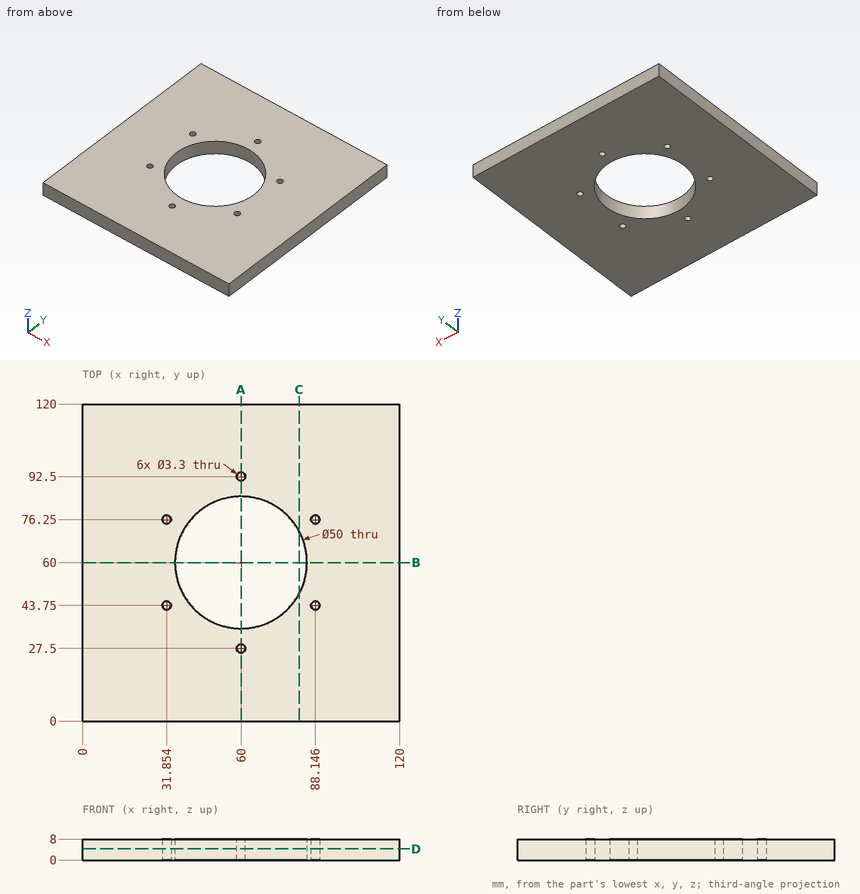
Here's the drawing with two shaded views (mm, measured from the low corner). I have some questions. Give positions to 0.01 mm unless a question says otherwise; leave off trailing zeros. Loops run counter-clockwise (first coordinate to the right, second up) from the corner with the lowest first, then second, coordinate; pieces in that order, holes last. Notation, with made-up numbers: M -9.75,78.25 L 30.25,78.25 A18 cw 30.25,102.25 Z; hole C 67,-2.5 d4. An arc over 180 degrees is marked long. Answer in a Markdown table with one row per item.
1. Suppose I cut it at D-D on z = 4.25. Write out the boundary of the cut face in (x, y).
Taken from the geometry:
| item | result |
|---|---|
| outline | M 0,0 L 120,0 L 120,120 L 0,120 Z; hole C 31.85,43.75 d3.3; hole C 31.85,76.25 d3.3; hole C 60,60 d50; hole C 60,27.5 d3.3; hole C 60,92.5 d3.3; hole C 88.15,43.75 d3.3; hole C 88.15,76.25 d3.3 |
2. If I drill on line 1 along X through (y, z) = (92.5, 1.25); line 2 along Y through (x, z) = (33, 5); line 3 along Y through (x, z) = (83, 3.75), over which ranges is the centre line in solid material (lowest first)?
Taken from the geometry:
| item | result |
|---|---|
| line 1 | x = 0 to 58.35, 61.65 to 120 |
| line 2 | y = 0 to 42.56, 44.94 to 75.06, 77.44 to 120 |
| line 3 | y = 0 to 50.2, 69.8 to 120 |
3. Suppose I cut it at A-A on x = 60. Write out the boundary of the cut face in (y, z).
Taken from the geometry:
| item | result |
|---|---|
| outline | M 0,0 L 25.85,0 L 25.85,8 L 0,8 Z; M 29.15,0 L 35,0 L 35,8 L 29.15,8 Z; M 85,0 L 90.85,0 L 90.85,8 L 85,8 Z; M 94.15,0 L 120,0 L 120,8 L 94.15,8 Z |
4. For pin 1 Ø2 at (x, y) = (60, 92.5) entering from +Z, with a flat end and sliding along its axis, tell me the tip position at first contact or that it passes through.
Taken from the geometry:
| item | result |
|---|---|
| pin 1 | passes through |
5. Suppose I cut it at C-C on x = 82. Write out the boundary of the cut face in (y, z).
Taken from the geometry:
| item | result |
|---|---|
| outline | M 0,0 L 48.13,0 L 48.13,8 L 0,8 Z; M 71.87,0 L 120,0 L 120,8 L 71.87,8 Z |
6. Suppose I cut it at B-B on y = 60. Write out the boundary of the cut face in (x, z).
Taken from the geometry:
| item | result |
|---|---|
| outline | M 0,0 L 35,0 L 35,8 L 0,8 Z; M 85,0 L 120,0 L 120,8 L 85,8 Z |
